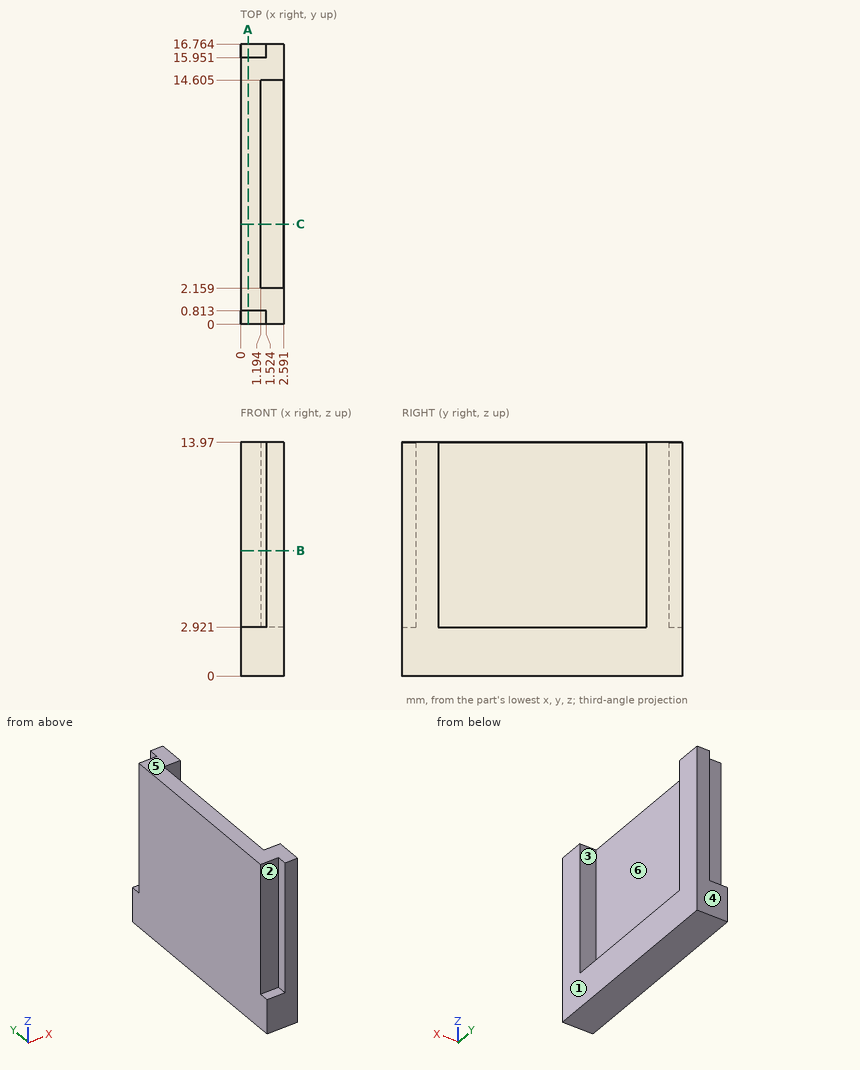
Input: dimensioned drawing with shaded views. Units: mm. Origin: part minimum x, y, z. A direction names the side the tool comes from. Coordinates: 2 decimals unless noted, no trailing zeros. Order: outer loops, then holes, each group sorted by start corner. A loop starts at its lowest first (then second) coordinate and runs counter-clockwise, first axis right, second up. Notation, with made-up numbers: (-18.5, -38) - (20.5, -38) arc R28 cw to (20.5, -12) - close; hole circle Ø9 at (32, 36). An arc over 180 degrees is marked (long way). One line per item, written item: value.
1) Cut plane A-A on x = 0.45. Output: boundary loops of the cut face in (y, z).
Computed values:
outline: (0, 0) - (16.76, 0) - (16.76, 2.92) - (15.95, 2.92) - (15.95, 13.97) - (0.81, 13.97) - (0.81, 2.92) - (0, 2.92) - close
2) Reachability of the marked faces 1, 2 and 3 from +Z, -Z, +X, -X, +Y, -Y: full face, straight path, thin tool, end or side. Return the list, or none.
Computed values:
face 1: +Z, -Z, +X, +Y, -Y
face 2: +Z, -X, -Y
face 3: +Z, +X
3) Cut plane C-C on y = 6. Output: boundary loops of the cut face in (x, z).
Computed values:
outline: (0, 0) - (2.59, 0) - (2.59, 2.92) - (1.19, 2.92) - (1.19, 13.97) - (0, 13.97) - close
4) Cut plane B-B on z = 7.5. Output: boundary loops of the cut face in (x, y) (1 decimal), plus the area to 3 significant figures.
Computed values:
outline: (0, 0.8) - (1.5, 0.8) - (1.5, 0) - (2.6, 0) - (2.6, 2.2) - (1.2, 2.2) - (1.2, 14.6) - (2.6, 14.6) - (2.6, 16.8) - (1.5, 16.8) - (1.5, 16) - (0, 16) - close
area: 23.6 mm^2
5) Contact query for flat-ended pins moving along their axis: pin 1 (1.2 mm diameter, centred on x = 0.5, z = 6.5, fed in from +Y); pin 2 (1 mm diameter, centred on y = 3, z = 11, fed in from +X). Output: stop coordinate, or through.
Computed values:
pin 1: stops at y = 15.95
pin 2: stops at x = 1.19
6) Mould query, pull axis Y, two halves, no side actions, for the marked faces 4, 5 and 6. Classes: released by +Y, released by -Y, zero draft, split by the parting line, or undercut.
Computed values:
face 4: released by +Y
face 5: zero draft
face 6: undercut
7) Ray query, line 1 (Y direction, x = 1.3, z = 8.5) (1 decimal); line 2 (Y direction, x = 2.35, z = 7.25) (3 decimals); line 3 (Z direction, x = 1.9, y = 3.5). Return the intervals inside material, ascending. Write a range as [from, to].
Computed values:
line 1: y = [0.8, 2.2], [14.6, 16]
line 2: y = [0, 2.159], [14.605, 16.764]
line 3: z = [0, 2.92]
